Part model, mm, in its own coordinate system. Round coordinates to 2 decimals unless told otherwise and drop trailing zeros. Order: outer loops, then holes, each group sorted by start corner. A loop starts at its lowest first (then second) coordinate and runs counter-clockwise, first axis right, second up. Notation, with made-up numbers: (-20, -33.5) -> (-14, -33.5) arc R27 cw to (-14, 2.5) -> close; hole circle Ø7 at (81, 32). An arc over 180 degrees is marked (long way). Answer as a JSON object with one key per item and string values. Group by question number.
```python
from build123d import *

# Parameters (mm, degrees)
F3_R      = 128.0515086977
F4_DEPTH  = 25.4
F5_R      = 35.56
F6_DEPTH  = 25.4
F7_R      = 28.702
F8_DEPTH  = 57.15
F10_DEPTH = 50.8
F11_R     = 5.079
F12_R     = 1.27
F13_R     = 2.54


# Not quite as in the source:
# - a fillet or chamfer is up to 0.001 mm smaller than in the source, because OpenCascade refuses the exact size


with BuildPart() as f1:
    # F0 (on Front) → F1 (revolve)
    with BuildSketch(Plane.XZ):
        with BuildLine():
            Line((0, 0), (0, -50.8))
            ThreePointArc((0, -50.8), (50.8, 0), (0, 50.8))
            Line((0, 50.8), (0, 0))
        make_face()
    revolve(axis=Axis((0, 0, 25.4), (0, 0, 1)))

    # F3 (on offset) → F4 (cut)
    with BuildSketch(Plane.XY.offset(-44.45)):
        with Locations((0, 3.5303835757)):
            Circle(F3_R)
    extrude(amount=-F4_DEPTH, mode=Mode.SUBTRACT)

    # F5 (on face) → F6 (join)
    with BuildSketch(Plane(origin=(0, 0, -44.45), x_dir=(1, 0, 0), z_dir=(0, 0, -1))):
        Circle(F5_R)
    extrude(amount=-F6_DEPTH)

    # F7 (on face) → F8 (cut)
    with BuildSketch(Plane(origin=(0, 0, -44.45), x_dir=(1, 0, 0), z_dir=(0, 0, -1))):
        Circle(F7_R)
    extrude(amount=-F8_DEPTH, mode=Mode.SUBTRACT)

    # F9 (on face) → F10 (cut)
    with BuildSketch(Plane(origin=(0, 0, -44.45), x_dir=(1, 0, 0), z_dir=(0, 0, -1))):
        with BuildLine():
            ThreePointArc((-5.08, 28.2488655347), (-2.5500848439, 28.588491938), (0, 28.702))
            Line((0, 28.702), (0, 32.0588655347))
            Line((0, 32.0588655347), (-5.08, 32.0588655347))
            Line((-5.08, 32.0588655347), (-5.08, 28.2488655347))
        make_face()
        with BuildLine():
            ThreePointArc((0, 28.702), (2.5500848439, 28.588491938), (5.08, 28.2488655347))
            Line((5.08, 28.2488655347), (5.08, 32.0588655347))
            Line((5.08, 32.0588655347), (0, 32.0588655347))
            Line((0, 32.0588655347), (0, 28.702))
        make_face()
        with BuildLine():
            Line((5.08, -32.0588655347), (5.08, -28.2488655347))
            ThreePointArc((5.08, -28.2488655347), (0, -28.702), (-5.08, -28.2488655347))
            Line((-5.08, -28.2488655347), (-5.08, -32.0588655347))
            Line((-5.08, -32.0588655347), (0, -32.0588655347))
            Line((0, -32.0588655347), (5.08, -32.0588655347))
        make_face()
    extrude(amount=-F10_DEPTH, mode=Mode.SUBTRACT)

    # F11 (radius 5.08 in the source; OpenCascade refuses exactly that, so slightly less here)
    f11_edges = [f1.edges().sort_by_distance(p)[0] for p in [
        (-5.08, -30.153866, 6.35),
        (5.08, -30.153866, 6.35),
        (5.08, 30.153866, 6.35),
        (-5.08, 30.153866, 6.35),
    ]]
    fillet(f11_edges, radius=F11_R)

    # F12
    f12_edges = [f1.edges().sort_by_distance(p)[0] for p in [
        (5.08, 28.248866, -21.5895),
        (5.08, 32.058866, -21.5895),
        (5.08, -32.058866, -21.5895),
        (5.08, -28.248866, -21.5895),
    ]]
    fillet(f12_edges, radius=F12_R)

    # F13
    f13_edges = [f1.edges().sort_by_distance(p)[0] for p in [
        (-28.702, 0, 12.7),
    ]]
    fillet(f13_edges, radius=F13_R)


solid = f1.part
```
Q1. Two-plate mould, pull along X, no slides. Class faces 1 (the cylindrical face through (-7.709, 34.714, -40.421)), 2 (the flat face through (29, -3, -44.45)), 3 (the cylindrical face through (-4.19, 30.22, 4.14)): +X half, -X half, draft (parallel to the pull), parting line (faces both ways), or undercut.
Q2. Band-saw the part on B-B (z = -0.5). List the corners of the cut face in (x, y).
Q3. Band-saw the part on D-D (x = -41). List the corners of the cut face in (y, z), plus the area to 3 significant figures.
Q4. Band-saw the part on A-A (y = 0). List the corners of the cut face in (x, z).
Q5. Band-saw the part on C-C (z = -28). List the corners of the cut face in (x, y).
Q6. Drop flat-ended pins along their axis: pin 1 Ø1 at (x, y) = (-18, -8.5) entering from -Z; pin 2 Ø1.6 at (y, z) = (30.5, -26.5) entering from +X; pin 3 Ø6 at (y, z) = (32, 2.5) entering from +X. Give the stop position or say it passes through.
Q7. Wall check: line 1 (Y direction, x = 17.5, z = -12.5); line 2 (Y direction, x = -13.5, z = -13); line 3 (X direction, y = 18, z = -40). Give the ranges that are in metal, low to high. Write a range as [from, to].
Completed:
{
 "1": {"face 1": "parting line", "face 2": "draft", "face 3": "undercut"},
 "2": {"outline": "circle Ø101.6 at (0, 0); hole (-6.08, -28.05) arc R1.27 cw to (-5.08, -29.29) -> (-5.08, -30.79) arc R1.27 ccw to (-3.81, -32.06) -> (3.81, -32.06) arc R1.27 ccw to (5.08, -30.79) -> (5.08, -29.29) arc R1.27 cw to (6.08, -28.05) arc R28.7 ccw to (6.08, 28.05) arc R1.27 cw to (5.08, 29.29) -> (5.08, 30.79) arc R1.27 ccw to (3.81, 32.06) -> (-3.81, 32.06) arc R1.27 ccw to (-5.08, 30.79) -> (-5.08, 29.29) arc R1.27 cw to (-6.08, 28.05) arc R28.7 ccw to start"},
 "3": {"outline": "circle Ø59.99 at (0, 0)", "area": "2,830 mm2"},
 "4": {"outline": "(-35.56, -44.45) -> (-28.7, -44.45) -> (-28.7, 10.16) arc R2.54 cw to (-26.16, 12.7) -> (26.16, 12.7) arc R2.54 cw to (28.7, 10.16) -> (28.7, -44.45) -> (35.56, -44.45) -> (35.56, -36.28) arc R50.8 ccw (long way) to (-35.56, -36.28) -> close"},
 "5": {"outline": "circle Ø84.77 at (0, 0); hole (-6.08, -28.05) arc R1.27 cw to (-5.08, -29.29) -> (-5.08, -30.79) arc R1.27 ccw to (-3.81, -32.06) -> (3.81, -32.06) arc R1.27 ccw to (5.08, -30.79) -> (5.08, -29.29) arc R1.27 cw to (6.08, -28.05) arc R28.7 ccw to (6.08, 28.05) arc R1.27 cw to (5.08, 29.29) -> (5.08, 30.79) arc R1.27 ccw to (3.81, 32.06) -> (-3.81, 32.06) arc R1.27 ccw to (-5.08, 30.79) -> (-5.08, 29.29) arc R1.27 cw to (-6.08, 28.05) arc R28.7 ccw to start"},
 "6": {"pin 1": "z = 12.7", "pin 2": "x = 31.81", "pin 3": "x = 41.64"},
 "7": {"line 1": "[-46.02, -22.75], [22.75, 46.02]", "line 2": "[-47.22, -25.33], [25.33, 47.22]", "line 3": "[-30.67, -22.36], [22.36, 30.67]"}
}
